```python
from build123d import *

# Parameters (mm, degrees)
BOSS_EXTRUDE1_DEPTH = 6.35
SKETCH2_R           = 1.5875
SKETCH2_W           = 80.264
SKETCH2_H           = 12.954
CUT_EXTRUDE1_DEPTH  = 162.484606465
SKETCH7_R           = 2.032
SKETCH7_W           = 49.149
SKETCH7_H           = 67.183
CUT_EXTRUDE4_DEPTH  = 162.484606465
SKETCH8_R           = 1.651
CUT_EXTRUDE5_DEPTH  = 162.484606465
CUT_EXTRUDE6_DEPTH  = 160.416662013
FILLET1_R           = 5.08
FILLET2_R           = 5.08
SKETCH10_R          = 1.651
CUT_EXTRUDE7_DEPTH  = 160.416662013


with BuildPart() as part:
    # Sketch1 → Boss-Extrude1 (new body)
    with BuildSketch(Plane(origin=(0, 0, 0), x_dir=(1, 0, 0), z_dir=(0, 1, 0))):
        with BuildLine():
            Line((-3.175, 112.5), (95.25, 112.5))
            Line((95.25, 112.5), (95.25, -112.5))
            Line((95.25, -112.5), (-3.175, -112.5))
            ThreePointArc((-3.175, -112.5), (-115.675, 0), (-3.175, 112.5))
        make_face()
    extrude(amount=-BOSS_EXTRUDE1_DEPTH)

    # Sketch2 → Cut-Extrude1 (cut, through all)
    with BuildSketch(Plane(origin=(0, 0, 0), x_dir=(1, 0, 0), z_dir=(0, 1, 0))):
        with Locations(Location((36.144045702, -66.3448, 0), (0, 0, 270))):
            Circle(SKETCH2_R)
        with Locations(Location((36.144045702, -59.9948, 0), (0, 0, 270))):
            Circle(SKETCH2_R)
        with Locations(Location((36.144045702, -53.6448, 0), (0, 0, 270))):
            Circle(SKETCH2_R)
        with Locations(Location((36.144045702, -47.2948, 0), (0, 0, 270))):
            Circle(SKETCH2_R)
        with Locations(Location((36.144045702, -40.9448, 0), (0, 0, 270))):
            Circle(SKETCH2_R)
        with Locations(Location((36.144045702, -34.5948, 0), (0, 0, 270))):
            Circle(SKETCH2_R)
        with Locations(Location((36.144045702, -28.2448, 0), (0, 0, 270))):
            Circle(SKETCH2_R)
        with Locations(Location((67.894045702, -66.3448, 0), (0, 0, 270))):
            Circle(SKETCH2_R)
        with Locations(Location((67.894045702, -59.9948, 0), (0, 0, 270))):
            Circle(SKETCH2_R)
        with Locations(Location((67.894045702, -53.6448, 0), (0, 0, 270))):
            Circle(SKETCH2_R)
        with Locations(Location((67.894045702, -47.2948, 0), (0, 0, 270))):
            Circle(SKETCH2_R)
        with Locations(Location((67.894045702, -40.9448, 0), (0, 0, 270))):
            Circle(SKETCH2_R)
        with Locations(Location((67.894045702, -34.5948, 0), (0, 0, 270))):
            Circle(SKETCH2_R)
        with Locations(Location((67.894045702, -28.2448, 0), (0, 0, 270))):
            Circle(SKETCH2_R)
        with Locations(Location((36.144045702, 66.3448, 0), (0, 0, 270))):
            Circle(SKETCH2_R)
        with Locations(Location((36.144045702, 59.9948, 0), (0, 0, 270))):
            Circle(SKETCH2_R)
        with Locations(Location((36.144045702, 53.6448, 0), (0, 0, 270))):
            Circle(SKETCH2_R)
        with Locations(Location((36.144045702, 47.2948, 0), (0, 0, 270))):
            Circle(SKETCH2_R)
        with Locations(Location((36.144045702, 40.9448, 0), (0, 0, 270))):
            Circle(SKETCH2_R)
        with Locations(Location((36.144045702, 34.5948, 0), (0, 0, 270))):
            Circle(SKETCH2_R)
        with Locations(Location((36.144045702, 28.2448, 0), (0, 0, 270))):
            Circle(SKETCH2_R)
        with Locations(Location((67.894045702, 66.3448, 0), (0, 0, 270))):
            Circle(SKETCH2_R)
        with Locations(Location((67.894045702, 59.9948, 0), (0, 0, 270))):
            Circle(SKETCH2_R)
        with Locations(Location((67.894045702, 53.6448, 0), (0, 0, 270))):
            Circle(SKETCH2_R)
        with Locations(Location((67.894045702, 47.2948, 0), (0, 0, 270))):
            Circle(SKETCH2_R)
        with Locations(Location((67.894045702, 40.9448, 0), (0, 0, 270))):
            Circle(SKETCH2_R)
        with Locations(Location((67.894045702, 34.5948, 0), (0, 0, 270))):
            Circle(SKETCH2_R)
        with Locations(Location((67.894045702, 28.2448, 0), (0, 0, 270))):
            Circle(SKETCH2_R)
        with Locations((52.019045702, -96.4438)):
            Rectangle(SKETCH2_W, SKETCH2_H)
        with Locations((52.019045702, 96.4438)):
            Rectangle(SKETCH2_W, SKETCH2_H)
    extrude(amount=-CUT_EXTRUDE1_DEPTH, mode=Mode.SUBTRACT)

    # Sketch7 → Cut-Extrude4 (cut, through all)
    with BuildSketch(Plane(origin=(0, 0, 0), x_dir=(1, 0, 0), z_dir=(0, 1, 0))):
        with Locations(Location((-40.297137944, 0, 0), (0, 0, 270))):
            Circle(SKETCH7_R)
        with Locations(Location((31.711862056, 0, 0), (0, 0, 270))):
            Circle(SKETCH7_R)
        with Locations(Location((82.511862056, 0, 0), (0, 0, 270))):
            Circle(SKETCH7_R)
        with Locations(Location((-40.297137944, 40.64, 0), (0, 0, 270))):
            Circle(SKETCH7_R)
        with Locations(Location((-40.297137944, -40.64, 0), (0, 0, 270))):
            Circle(SKETCH7_R)
        with Locations((-3.022637944, 0)):
            Rectangle(SKETCH7_W, SKETCH7_H)
    extrude(amount=-CUT_EXTRUDE4_DEPTH, mode=Mode.SUBTRACT)

    # Sketch8 → Cut-Extrude5 (cut, through all)
    with BuildSketch(Plane(origin=(0, 0, 0), x_dir=(1, 0, 0), z_dir=(0, 1, 0))):
        with Locations(Location((-100.5586, 33.02, 0), (0, 0, 270))):
            Circle(SKETCH8_R)
        with Locations(Location((-100.5586, -33.02, 0), (0, 0, 270))):
            Circle(SKETCH8_R)
        with Locations(Location((-75.1586, 33.02, 0), (0, 0, 270))):
            Circle(SKETCH8_R)
        with Locations(Location((-75.1586, -33.02, 0), (0, 0, 270))):
            Circle(SKETCH8_R)
        with BuildLine():
            Line((-90.2716, 25.4), (-229.776686608, 25.4))
            Line((-229.776686608, 25.4), (-229.776686608, -25.4))
            Line((-229.776686608, -25.4), (-90.2716, -25.4))
            ThreePointArc((-90.2716, -25.4), (-64.8716, 0), (-90.2716, 25.4))
        make_face()
    extrude(amount=-CUT_EXTRUDE5_DEPTH, mode=Mode.SUBTRACT)

    # Sketch9 → Cut-Extrude6 (cut, through all)
    with BuildSketch(Plane(origin=(0, 0, 0), x_dir=(1, 0, 0), z_dir=(0, 1, 0))):
        Polygon((-105.15131959, 47.508738596), (-16.481779133, 71.267670354), (15.119014667, 149.482379647), (-15.990379699, 149.482379647), (-132.083987526, 149.482379647), (-132.083987526, 47.508738596), align=None)
        Polygon((-105.15131959, -47.508738596), (-16.481779133, -71.267670354), (15.119014667, -149.482379647), (-132.083987526, -149.482379647), (-132.083987526, -47.508738596), align=None)
    extrude(amount=-CUT_EXTRUDE6_DEPTH, mode=Mode.SUBTRACT)

    # Fillet1
    fillet1_edges = [part.edges().sort_by_distance(p)[0] for p in [
        (0.177163396, -3.175, -112.5),
    ]]
    fillet(fillet1_edges, radius=FILLET1_R)

    # Fillet2
    fillet2_edges = [part.edges().sort_by_distance(p)[0] for p in [
        (0.177163396, -3.175, 112.5),
        (95.25, -3.175, -112.5),
        (95.25, -3.175, 112.5),
    ]]
    fillet(fillet2_edges, radius=FILLET2_R)

    # Sketch10 → Cut-Extrude7 (cut, through all)
    with BuildSketch(Plane(origin=(0, 0, 0), x_dir=(1, 0, 0), z_dir=(0, 1, 0))):
        with Locations(Location((-91.401386068, 41.91, 0), (0, 0, 270))):
            Circle(SKETCH10_R)
        with Locations(Location((-79.134128074, 45.197001873, 0), (0, 0, 270))):
            Circle(SKETCH10_R)
        with Locations(Location((-66.434128074, 45.197001873, 0), (0, 0, 270))):
            Circle(SKETCH10_R)
        with Locations(Location((-54.16687008, 48.484003746, 0), (0, 0, 270))):
            Circle(SKETCH10_R)
        with Locations(Location((-43.57652014, 55.493603459, 0), (0, 0, 270))):
            Circle(SKETCH10_R)
        with Locations(Location((-30.87652014, 55.493603459, 0), (0, 0, 270))):
            Circle(SKETCH10_R)
        with Locations(Location((-32.363085711, 49.531314612, 0), (0, 0, 270))):
            Circle(SKETCH10_R)
        with Locations(Location((-27.437235207, 42.658017348, 0), (0, 0, 270))):
            Circle(SKETCH10_R)
        with Locations(Location((-15.169977213, 45.94501922, 0), (0, 0, 270))):
            Circle(SKETCH10_R)
        with Locations(Location((-2.902719219, 49.232021093, 0), (0, 0, 270))):
            Circle(SKETCH10_R)
        with Locations(Location((9.364538775, 52.519022966, 0), (0, 0, 270))):
            Circle(SKETCH10_R)
        with Locations(Location((-8.367598507, 67.98932858, 0), (0, 0, 270))):
            Circle(SKETCH10_R)
        with Locations(Location((-3.61009477, 79.764563533, 0), (0, 0, 270))):
            Circle(SKETCH10_R)
        with Locations(Location((4.032956024, 89.907234511, 0), (0, 0, 270))):
            Circle(SKETCH10_R)
        with Locations(Location((-91.401386068, -41.91, 0), (0, 0, 270))):
            Circle(SKETCH10_R)
        with Locations(Location((-79.134128074, -45.197001873, 0), (0, 0, 270))):
            Circle(SKETCH10_R)
        with Locations(Location((-66.434128074, -45.197001873, 0), (0, 0, 270))):
            Circle(SKETCH10_R)
        with Locations(Location((-54.16687008, -48.484003746, 0), (0, 0, 270))):
            Circle(SKETCH10_R)
        with Locations(Location((-43.57652014, -55.493603459, 0), (0, 0, 270))):
            Circle(SKETCH10_R)
        with Locations(Location((-30.87652014, -55.493603459, 0), (0, 0, 270))):
            Circle(SKETCH10_R)
        with Locations(Location((-32.363085711, -49.531314612, 0), (0, 0, 270))):
            Circle(SKETCH10_R)
        with Locations(Location((-27.438316181, -42.662051597, 0), (0, 0, 270))):
            Circle(SKETCH10_R)
        with Locations(Location((-15.171058187, -45.94905347, 0), (0, 0, 270))):
            Circle(SKETCH10_R)
        with Locations(Location((-2.903800193, -49.236055343, 0), (0, 0, 270))):
            Circle(SKETCH10_R)
        with Locations(Location((9.363457801, -52.523057216, 0), (0, 0, 270))):
            Circle(SKETCH10_R)
        with Locations(Location((-8.367598507, -67.98932858, 0), (0, 0, 270))):
            Circle(SKETCH10_R)
        with Locations(Location((-3.61009477, -79.764563533, 0), (0, 0, 270))):
            Circle(SKETCH10_R)
        with Locations(Location((4.032956024, -89.907234511, 0), (0, 0, 270))):
            Circle(SKETCH10_R)
    extrude(amount=-CUT_EXTRUDE7_DEPTH, mode=Mode.SUBTRACT)


solid = part.part
```
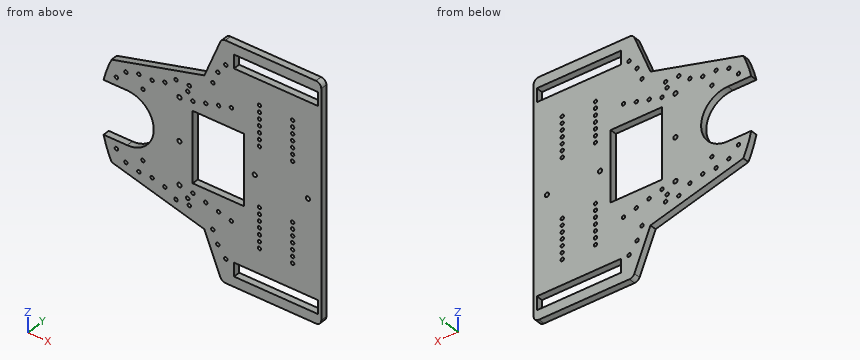
The listing builds one solid part. Answer for the finished solid, in the listing's coordinates (mm). Round coordinates to 2 decimals unless told otherwise and drop trailing zeros. Write each loop counter-clockwise with the first axis right and the second up, starting at its lowest first coordinate (ties: lowest second). Pieces come first, ordered by that corner, then holes. Notation, with made-up numbers: (-27.5, 59) -> (-18.5, 59) arc R29 cw to (-18.5, 87) -> close; hole circle Ø2 at (61.25, 3.25). An arc over 180 degrees is marked (long way). Answer as a JSON object with one key per item and string values. Group by question number.
Q1. Each of these flat-tipped pins is pushed along its axis until it touches: pin 1 Ø2 at (y, z) = (-5, -80) entering from -X; pin 2 Ø1.9 at (x, z) = (67.89, -40.94) entering from +Y; pin 3 Ø1.5 at (x, y) = (-81, -4.5) entering from +Z; pin 4 Ø1.9 at (y, z) = (-4, 94.5) entering from -X. Where does it stop, or does it pass through?
Q2. Section B-B (z = -11) is taken. Write down the section's boundary in (x, y).
Q3. Section A-A (x = 15.5) is taken. Write down the section's boundary in (y, z), plus the area to 3 significant figures.
Q4. Straight lines are drawn through the part: line 1 along Z through (x, y) = (4, -6); line 2 along Z through (x, y) = (34, -0.5); line 3 along Z through (x, y) = (19, -5.5). For each, find the intervals that lie inside material, in ascending order.
Q5. Section C-C (x = -96) is taken. Write down the section's boundary in (y, z).
Q6. Section D-D (y = -2.5) is taken. Count the separate pieces of the cut face and the enclosed holes in it, plus the area to 3 significant figures.
Check values:
{
 "1": {"pin 1": "x = -13.36", "pin 2": "through", "pin 3": "z = 54.18", "pin 4": "x = -7.48"},
 "2": {"outline": "(-67.38, -6.35) -> (-27.6, -6.35) -> (-27.6, 0) -> (-67.38, 0) -> close; (21.55, -6.35) -> (95.25, -6.35) -> (95.25, 0) -> (21.55, 0) -> close"},
 "3": {"outline": "(-6.35, -112.5) -> (0, -112.5) -> (0, -102.92) -> (-6.35, -102.92) -> close; (-6.35, -89.97) -> (0, -89.97) -> (0, -33.59) -> (-6.35, -33.59) -> close; (-6.35, 33.59) -> (0, 33.59) -> (0, 89.97) -> (-6.35, 89.97) -> close; (-6.35, 102.92) -> (0, 102.92) -> (0, 112.5) -> (-6.35, 112.5) -> close", "area": "838 mm^2"},
 "4": {"line 1": "-112.5 to -91.56, -88.26 to -33.59, 33.59 to 88.26, 91.56 to 112.5", "line 2": "-112.5 to -102.92, -89.97 to 89.97, 102.92 to 112.5", "line 3": "-112.5 to -102.92, -89.97 to -33.59, 33.59 to 89.97, 102.92 to 112.5"},
 "5": {"outline": "(-6.35, -49.96) -> (0, -49.96) -> (0, -25.4) -> (-6.35, -25.4) -> close; (-6.35, 25.4) -> (0, 25.4) -> (0, 49.96) -> (-6.35, 49.96) -> close"},
 "6": {"separate pieces": "1", "enclosed holes": "68", "area": "27,400 mm^2"}
}
